```python
from build123d import *

# Parameters (mm, degrees)
F0_W     = 34.5
F0_H     = 19.2
F1_DEPTH = 16.4
F2_W     = 11.3
F2_H     = 11.3
F3_DEPTH = 11.3
F4_R     = 1
F5_R     = 2


with BuildPart() as f1:
    # F0 (on Top) → F1 (new body)
    with BuildSketch(Plane.XY):
        with Locations((17.25, 9.6)):
            Rectangle(F0_W, F0_H)
    extrude(amount=F1_DEPTH)

    # F2 (on face) → F3 (cut)
    with BuildSketch(Plane.XY.offset(16.4)):
        with Locations((5.65, 13.55)):
            Rectangle(F2_W, F2_H)
    extrude(amount=-F3_DEPTH, mode=Mode.SUBTRACT)

    # F4
    f4_edges = [f1.edges().sort_by_distance(p)[0] for p in [
        (34.5, 0, 8.2),
        (34.5, 9.6, 0),
        (17.25, 0, 0),
    ]]
    fillet(f4_edges, radius=F4_R)

    # F5
    f5_edges = [f1.edges().sort_by_distance(p)[0] for p in [
        (0, 19.2, 2.55),
        (0, 3.95, 16.4),
        (22.9, 19.2, 16.4),
    ]]
    fillet(f5_edges, radius=F5_R)


solid = f1.part
```
CAD build for the part. Positions are in the model's coordinates, mm. A direction names the side the tool comes from. Give positions to 0.01 mm unless a question says otherwise; leave off trailing zeros. Write each loop counter-clockwise with the first axis right and the second up, starting at its lowest first coordinate (ties: lowest second). Pieces come first, ordered by that corner, then holes. Notation, with made-up numbers: (-16.5, 76.25) -> (8.5, 76.25) arc R14 cw to (8.5, 96.25) -> close; hole circle Ø8 at (49.25, -14). An arc over 180 degrees is marked (long way). Write each question's results on one line, items separated by ' | '.
1. Which spindle directions (+Z, -Z, +X, -X, +Y, -Y) get a long thin tool onto all of the face, cutting with end or side? Do faces 1 (the cylindrical face through (16.984, 0.301, 0.285)), 2 (the flat face through (6, 14, 5.1)). Say none if no direction does.
Geometry check:
face 1: -Z, +X, -X, -Y | face 2: +Z, -X, +Y
2. Drop flat-ended pins along their axis: P1, Ø9, axis at x = 4.5, y = 13.5, coming from the +Z side; P2, Ø3.5, axis at x = 4.5, z = 12.5, coming from the +Y side. Give the stop position or say it passes through.
Geometry check:
P1: z = 5.1 | P2: y = 7.9
3. Wall check: probe 1 along Z at (x, y) = (9, 13.25); probe 2 along Y at (x, z) = (11, 14.25); probe 3 along X at (y, z) = (16.75, 6.25). Give the ranges that are in metal, low to high. Write a range as [from, to].
Geometry check:
probe 1: [0, 5.1] | probe 2: [0, 7.9] | probe 3: [11.3, 34.5]
4. Cut at B-B, the plane y = 18. Write the cut outline in (x, z).
Geometry check:
outline: (0.17, 0) -> (33.5, 0) arc R1 ccw to (34.5, 1) -> (34.5, 16.23) -> (11.3, 16.23) -> (11.3, 5.1) -> (0.17, 5.1) -> close
5. Cut at A-A, the plane x = 5. Write the cut outline in (y, z), then the cut area to 3 significant figures.
Geometry check:
outline: (0, 1) arc R1 ccw to (1, 0) -> (19.2, 0) -> (19.2, 5.1) -> (7.9, 5.1) -> (7.9, 16.4) -> (0, 16.4) -> close | area: 187 mm²
